Autodesk Inventor part; units mm, degrees
ref_plane "YZ Plane" through (0, 0, 0) normal (1, 0, 0) x (0, 1, 0)
ref_plane "XZ Plane" through (0, 0, 0) normal (0, 1, 0) x (-1, 0, 0)
ref_plane "XY Plane" through (0, 0, 0) normal (0, 0, 1) x (1, 0, 0)
sketch "Sketch1" plane through (0, 0, 0) normal (0, 1, 0) x (-1, 0, 0)
  line L0 (-33.3375, 17.4625) -> (33.3375, 17.4625)
  line L1 (42.8625, 7.9375) -> (42.8625, -7.9375)
  line L2 (33.3375, -17.4625) -> (-33.3375, -17.4625)
  line L3 (-42.8625, -7.9375) -> (-42.8625, 7.9375)
  arc A0 (-42.8625, 7.9375) -> (-33.3375, 17.4625) centre (-42.8625, 17.4625) ccw
  arc A1 (-33.3375, -17.4625) -> (-42.8625, -7.9375) centre (-42.8625, -17.4625) ccw
  arc A2 (42.8625, -7.9375) -> (33.3375, -17.4625) centre (42.8625, -17.4625) ccw
  arc A3 (33.3375, 17.4625) -> (42.8625, 7.9375) centre (42.8625, 17.4625) ccw
  circle A4 centre (-39.6875, -4.7625) radius 1.5875
  line L4 (0, 15.213) -> (0, -8.9791)
  circle A5 centre (39.6875, -4.7625) radius 1.5875
  line L5 (-13.6455, 0) -> (11.519, 0)
  circle A6 centre (-39.6875, 4.7625) radius 1.5875
  circle A7 centre (39.6875, 4.7625) radius 1.5875
  line L6 (-42.8625, -13.6689) -> (-42.8625, -17.4625)
  line L7 (-42.8625, -17.4625) -> (-40.918, -17.4625)
  circle A8 centre (6.0427, 12.8524) radius 0.9004
  circle A9 centre (13.6423, 12.8524) radius 0.9004
  circle A10 centre (-6.0427, 12.8524) radius 0.9004
  circle A11 centre (-13.6423, 12.8524) radius 0.9004
  circle A12 centre (20.6375, 11.1125) radius 1.27
  circle A13 centre (27.6225, 11.1125) radius 1.27
  circle A14 centre (-9.8425, 5.0546) radius 0.4001
  circle A15 centre (9.8425, 5.0546) radius 0.4001
  circle A16 centre (3.4798, 4.1021) radius 0.6502
  circle A17 centre (-6.0198, -12.9972) radius 0.6502
  circle A18 centre (-6.0198, 2.2022) radius 0.6502
  circle A19 centre (3.4798, -14.8971) radius 0.6502
  line L8 (-13.6423, 12.8524) -> (-6.0427, 12.8524)
  point P0 (0, 0)
  dimension "d3" = 17.4625
  dimension "d4" = 42.8625
  dimension "d5" = 19.05
  dimension "d6" = 19.05
  dimension "d7" = 19.05
  dimension "d8" = 19.05
  dimension "d9" = 85.725
  dimension "d11" = 85.725
  dimension "d12" = 85.725
  dimension "d13" = 17.4625
  dimension "d14" = 17.4625
  dimension "d15" = 42.8625
  dimension "d19" = 34.925
  dimension "d20" = 42.8625
  dimension "d22" = 17.4625
  dimension "d23" = 42.8625
  dimension "d26" = 39.6875
  dimension "d27" = 3.175
  dimension "d28" = 4.7625
  dimension "d29" = 42.8625
  dimension "d30" = 17.4625
  dimension "d31" = 42.8625
  dimension "d32" = 34.925
  dimension "d33" = 1.8009
  dimension "d34" = 48.9052
  dimension "d35" = 30.3149
  dimension "d36" = 1.8009
  dimension "d37" = 1.8009
  dimension "d38" = 1.8009
  dimension "d39" = 30.3149
  dimension "d40" = 30.3149
  dimension "d41" = 30.3149
  dimension "d42" = 29.2202
  dimension "d43" = 36.8198
  dimension "d45" = 6.0427
  dimension "d46" = 6.0427
  dimension "d47" = 2.54
  dimension "d48" = 2.54
  dimension "d49" = 63.5
  dimension "d50" = 70.485
  dimension "d51" = 28.575
  dimension "d52" = 28.575
  dimension "d53" = 0.8001
  dimension "d54" = 0.8001
  dimension "d55" = 33.02
  dimension "d56" = 52.705
  dimension "d57" = 22.5171
  dimension "d58" = 22.5171
  dimension "d59" = 1.3005
  dimension "d61" = 21.5646
  dimension "d62" = 1.3005
  dimension "d63" = 1.3005
  dimension "d64" = 1.3005
  dimension "d65" = 36.8427
  dimension "d66" = 19.6647
  dimension "d67" = 36.8427
  dimension "d68" = 4.4653
  dimension "d69" = 46.3423
  dimension "d70" = 2.5654
  dimension "d73" = 56.5048
  dimension "d74" = 7.5997
  dimension "d75" = 7.5997
  dimension "d76" = 19.685
  dimension "d77" = 46.3423
extrude "Extrusion2" add sketch "Sketch1" along normal blind 1.5748
properties part number "pcb"
For this review, take the finished solid that the model builds, in its own axes (mm). Round coordinates to 2 decimals unless told otherwise and drop trailing zeros. Write each loop counter-clockwise with the first axis right and the second up, starting at its lowest first coordinate (ties: lowest second). Pieces come first, ordered by that corner, then holes. Notation, with made-up numbers: (-36, -22) - (-29, -22) arc R14 ccw to (-29, 5) - close; hole circle Ø10 at (78.5, 17). An arc over 180 degrees is marked (long way). Write each question's results on one line, items separated by ' | '.
Item 1: Take a section at A-A on x = 13.5. State the section outline as (y, z) points, then the cut area to 3 significant figures.
Calculated:
outline: (0, -17.46) - (1.57, -17.46) - (1.57, 11.96) - (0, 11.96) - close; (0, 13.74) - (1.57, 13.74) - (1.57, 17.46) - (0, 17.46) - close | area: 52.2 mm^2
Item 2: Take a section at B-B on y = 1.2. Count the separate pieces of the cut face and the enclosed holes in it, then the cut area to 3 significant figures.
Calculated:
separate pieces: 1 | enclosed holes: 16 | area: 2,650 mm^2
Item 3: Take a section at D-D on z = 15. State the section outline as (x, y) points, then the cut area to 3 significant figures.
Calculated:
outline: (-33.66, 0) - (33.66, 0) - (33.66, 1.57) - (-33.66, 1.57) - close | area: 106 mm^2
Item 4: Take a section at C-C on x = -34.5. State the section outline as (y, z) points.
Calculated:
outline: (0, -12.9) - (1.57, -12.9) - (1.57, 12.9) - (0, 12.9) - close
Item 5: Draft analysis for pull direction X (two halves, no side actions). For faces 1 (the face through (36.202, 0.776, -10.654)), 2 (the face through (0, 1, -17.462)), 3 (the face through (6.16, 0.78, 11.96)), state which applies: pulls with the +X half, pulls with the -X half, needs draft (parallel to the pull), parting line crosses it, or undercut.
Calculated:
face 1: pulls with the +X half | face 2: needs draft | face 3: undercut
Item 6: To check wall thickness, follow line 1 along Z through (x, y) = (6, 1.2); line 2 along X through (y, z) = (0.15, -5); line 3 along Z through (x, y) = (-13.5, 1.25). State the ranges of each line that lie inside material, in increasing order. Write a range as from..to.
Calculated:
line 1: z = -17.46..-13.65, -12.35..1.55, 2.85..11.95, 13.75..17.46 | line 2: x = -42.86..-41.26, -38.12..38.12, 41.26..42.86 | line 3: z = -17.46..11.96, 13.74..17.46
